Build history of the part. All positions in model axes, mm. A direction names the side the tool comes from. Coordinates: 2 decimals unless noted, no trailing zeros. Loops run counter-clockwise (first coordinate to the right, second up) from the corner with the lowest first, then second, coordinate; pieces in that order, holes last.
Item 1: Mould opens along Z. For faces 1 (the face through (6, 8.5, -2)), 2 (the face through (0.33, 0.74, 7.493)), 3 (the face through (2.44, 5.07, 0.54)) say: released by +Z, released by -Z, zero draft, split by the parting line, or undercut.
Item 2: Flat gauge pins, fed straight in: pin 1 (3 mm diameter, centred on x = 0, z = 0, fed in from -Y); pin 2 (1.5 mm diameter, centred on y = 6.5, z = 2.5, fed in from +X). Where does each tip first touch, or does it go through?
Item 3: 3-axis set-ups, long thin cutter, end or side, ignore diameter. For faces 4 (the face through (-2, 0, 2)), 5 (the face through (0.268, 4.951, 6.094)): which of +Z, -Z, +X, -X, +Y, -Y reach the whole face in a straight line?
Item 4: Drill centre lines: line 1 along X through (y, z) = (3.25, 0); line 2 along Y through (x, z) = (5, -4.75). Where is each one in solid material? Low to high.
Item 5: Cut at C-C (z = -3.5). List the corners of the cut face in (x, y), and give its area (3 significant figures).
Item 6: Cut at B-B (z = 0). List the corners of the cut face in (x, y).
Item 7: Cut at D-D (y = 5.25). List the corners of the cut face in (x, z).
Item 8: Cut at A-A (x = 0). List the corners of the cut face in (y, z), and give its area (3 significant figures).
Autodesk Inventor part; units mm, degrees
ref_plane "YZ Plane" through (0, 0, 0) normal (1, 0, 0) x (0, 1, 0)
ref_plane "XZ Plane" through (0, 0, 0) normal (0, 1, 0) x (-1, 0, 0)
ref_plane "XY Plane" through (0, 0, 0) normal (0, 0, 1) x (1, 0, 0)
sketch "Sketch1" plane through (0, 0, 0) normal (1, 0, 0) x (0, 1, 0)
  line L0 (0, 0) -> (17.2785, 0)
  line L1 (0, -2.5) -> (10, -2.5)
  line L2 (10, -2.5) -> (10, -7.5)
  line L3 (10, -7.5) -> (8.5, -7.5)
  line L4 (8.5, -7.5) -> (8.5, -6.1)
  line L5 (8.5, -6.1) -> (1.5, -6.1)
  line L6 (1.5, -6.1) -> (1.5, -7.5)
  line L7 (1.5, -7.5) -> (0, -7.5)
  line L8 (0, -7.5) -> (0, -2.5)
  point P0 (5, -2.5)
  dimension "d1" = 5
  dimension "d2" = 15
  dimension "d3" = 12.2
  dimension "d4" = 7
  dimension "d5" = 1.5
revolve "Revolution1" add sketch "Sketch1" angle 360 about axis through (0, 0, 0) along (0, 1, 0)
properties part number "6mm toothed idler" material "Aluminum 6061"
Filled sheet:
1. face 1: zero draft
1. face 2: split by the parting line
1. face 3: undercut
2. pin 1: passes through
2. pin 2: stops at x = 5.84
3. face 4: +Z, -Z, +X, -X, -Y
3. face 5: none
4. line 1: x = -6.1 to -2.5, 2.5 to 6.1
4. line 2: y = 0 to 1.5, 8.5 to 10
5. outline: (-6.63, 0) - (6.63, 0) - (6.63, 1.5) - (5, 1.5) - (5, 8.5) - (6.63, 8.5) - (6.63, 10) - (-6.63, 10) - (-6.63, 8.5) - (-5, 8.5) - (-5, 1.5) - (-6.63, 1.5) - close
5. area: 110 mm2
6. outline: (-7.5, 0) - (-2.5, 0) - (-2.5, 10) - (-7.5, 10) - (-7.5, 8.5) - (-6.1, 8.5) - (-6.1, 1.5) - (-7.5, 1.5) - close; (2.5, 0) - (7.5, 0) - (7.5, 1.5) - (6.1, 1.5) - (6.1, 8.5) - (7.5, 8.5) - (7.5, 10) - (2.5, 10) - close
7. outline: circle Ø12.2 at (0, 0); hole circle Ø5 at (0, 0)
8. outline: (0, -7.5) - (1.5, -7.5) - (1.5, -6.1) - (8.5, -6.1) - (8.5, -7.5) - (10, -7.5) - (10, -2.5) - (0, -2.5) - close; (0, 2.5) - (10, 2.5) - (10, 7.5) - (8.5, 7.5) - (8.5, 6.1) - (1.5, 6.1) - (1.5, 7.5) - (0, 7.5) - close
8. area: 80.4 mm2
